Here's how the part is built. I have some questions about the finished solid (model axes, mm). A direction names the side the tool comes from. Round coordinates to 2 decimals unless told otherwise and drop trailing zeros. Order: outer loops, then holes, each group sorted by start corner. A loop starts at its lowest first (then second) coordinate and runs counter-clockwise, first axis right, second up. Notation, with made-up numbers: M -39,81 L 5,81 A23 cw 5,115 Z; hole C -13,52.5 d10. An arc over 180 degrees is marked long. Answer as CSV lines item,"result". Start each with the question number.
```python
from build123d import *

# Parameters (mm, degrees)
F0_R     = 18.25
F1_DEPTH = 1
F2_DEPTH = 10
F3_R     = 2


with BuildPart() as f1:
    # F0 (on Top) → F1 (new body)
    with BuildSketch(Plane.XY):
        Circle(F0_R)
        with BuildLine():
            ThreePointArc((15.0684210526, -1.9956670515), (-15.1670695917, -1), (14.6759622394, 3.9567830807))
            ThreePointArc((14.6759622394, 3.9567830807), (16.6541844606, 3.2144182213), (16.8625088904, 1.1117842368))
            ThreePointArc((16.8625088904, 1.1117842368), (16.9320508076, -1), (15.0684210526, -1.9956670515))
        make_face(mode=Mode.SUBTRACT)
        with BuildLine():
            ThreePointArc((16.8625088904, 1.1117842368), (16.6541844606, 3.2144182213), (14.6759622394, 3.9567830807))
            ThreePointArc((14.6759622394, 3.9567830807), (-15.1670695917, -1), (15.0684210526, -1.9956670515))
            ThreePointArc((15.0684210526, -1.9956670515), (16.9320508076, -1), (16.8625088904, 1.1117842368))
        make_face()
    extrude(amount=-F1_DEPTH)

    # F0 (on Top) → F2 (join)
    with BuildSketch(Plane.XY):
        Circle(F0_R)
        with BuildLine():
            ThreePointArc((15.0684210526, -1.9956670515), (-15.1670695917, -1), (14.6759622394, 3.9567830807))
            ThreePointArc((14.6759622394, 3.9567830807), (16.6541844606, 3.2144182213), (16.8625088904, 1.1117842368))
            ThreePointArc((16.8625088904, 1.1117842368), (16.9320508076, -1), (15.0684210526, -1.9956670515))
        make_face(mode=Mode.SUBTRACT)
    extrude(amount=F2_DEPTH)

    # F3
    f3_edges = [f1.edges().sort_by_distance(p)[0] for p in [
        (-18.25, 0, -1),
    ]]
    fillet(f3_edges, radius=F3_R)


solid = f1.part
```
Item 1: If we section it at A-A on z = 6: Please give me the cut outline in (x, y).
Item 2: For P1, Ø2, axis at x = -8.5, z = 2, coming from the -Y side; P2, Ø5, axis at x = 14, z = 4.5, coming from the -Y side; P3, Ø1, axis at x = -2.5, y = -8.5, coming from the +Z side, each with a flat end and sliding along its axis, tell me the tip position at first contact or that it passes through.
Item 3: If I drill on line 1 along X through (y, z) = (0, 5.75); line 2 along Y through (x, z) = (0, 2); line 3 along Z through (x, y) = (4, 11), over which ranges is the centre line in solid material (lowest first)?
Item 4: Which directions (+Z, -Z, +X, -X, +Y, -Y) give clear straight access to the entire face, cutting with the end or side of a thin tool? Please do faces 4 (the flat face through (1, 0, 0)), 5 (the flat face through (-11, -11, 10)).
Item 5: We'd pull the mould along Y, two halves only. Please class faces 1 (the cylindrical face through (-3.956, -17.816, 5.437)), 2 (the cylindrical face through (16.635, 3.239, 4.93)), 3 (the flat face through (0, 0, -1)): pulls with the +Y half, pulls with the -Y half, needs draft (parallel to the pull), parting line crosses it, or undercut.
Geometry says:
1,outline,"C 0,0 d36.5; hole M 14.68,3.96 A15.2 ccw long 15.07,-2 A2 ccw 16.86,1.11 A2 ccw Z"
2,P1,"y = -16.64"
2,P2,"y = -14.17"
2,P3,"z = 0"
3,line 1,"-18.25 to -15.2, 17.2 to 18.25"
3,line 2,"-18.25 to -15.2, 15.2 to 18.25"
3,line 3,"-1 to 0"
4,face 4,"+Z"
4,face 5,"+Z, +X, -X, +Y, -Y"
5,face 1,"parting line crosses it"
5,face 2,"undercut"
5,face 3,"needs draft"
